CAD build for the part. Positions are in the model's coordinates, mm. A direction names the side the tool comes from. Give positions to 0.01 mm unless a question says otherwise; leave off trailing zeros. Loops run counter-clockwise (first coordinate to the right, second up) from the corner with the lowest first, then second, coordinate; pieces in that order, holes last. Notation, with made-up numbers: (-10, 64) -> (-4, 64) arc R24 cw to (-4, 79) -> close; hole circle Ø10 at (-2.5, -34). An arc over 180 degrees is marked (long way). Use one line per item in the form item = value.
Autodesk Inventor part; units mm, degrees
ref_plane "YZ Plane" through (0, 0, 0) normal (1, 0, 0) x (0, 1, 0)
ref_plane "XZ Plane" through (0, 0, 0) normal (0, 1, 0) x (-1, 0, 0)
ref_plane "XY Plane" through (0, 0, 0) normal (0, 0, 1) x (1, 0, 0)
sketch "MainSketch1" plane through (0, 0, 0) normal (0, 0, 1) x (1, 0, 0)
  line L0 (0, 0) -> (86.36, 0)
  line L1 (86.36, 0) -> (86.36, 25.4)
  line L2 (86.36, 25.4) -> (76.2, 25.4)
  line L3 (76.2, 25.4) -> (76.2, 19.05)
  line L4 (76.2, 19.05) -> (67.31, 19.05)
  line L5 (67.31, 19.05) -> (67.31, 25.4)
  line L6 (67.31, 25.4) -> (19.05, 25.4)
  line L7 (19.05, 25.4) -> (19.05, 19.05)
  line L8 (19.05, 19.05) -> (10.16, 19.05)
  line L9 (10.16, 19.05) -> (10.16, 25.4)
  line L10 (10.16, 25.4) -> (0, 25.4)
  line L11 (0, 25.4) -> (0, 0)
  line L12 (381, 0) -> (381, 63.5) construction
  dimension "d0" = 86.36
  dimension "d1" = 10.16
  dimension "d2" = 19.05
  dimension "d3" = 67.31
  dimension "d4" = 76.2
  dimension "d5" = 19.05
  dimension "d6" = 25.4
  dimension "d7" = 25.4
  dimension "d8" = 19.05
  dimension "d9" = 25.4
  dimension "d10" = 381
  dimension "d30" = 63.5
revolve "MainRevolution1" add sketch "MainSketch1" angle 45 about axis through (381, 0, 0) along (0, 1, 0)
sketch "HeadSketch" plane through (19.05, 25.4, 0) normal (0, 1, 0) x (1, 0, 0)
  line L0 (48.26, 0) -> (0, 0)
  arc A0 (31.75, 9.3356) -> (16.51, 9.3356) centre (24.13, 25.4) ccw
  arc A1 (-19.05, 0) -> (92.5423, -269.4077) centre (361.95, 0) ccw
  arc A2 (67.31, 0) -> (153.6081, -208.3419) centre (361.95, 0) ccw
  line L1 (-8.89, 0) -> (-19.05, 0)
  line L2 (67.31, 0) -> (57.15, 0)
  line L3 (57.15, 0) -> (48.26, 0)
  line L4 (0, 0) -> (-8.89, 0)
  line L5 (92.5423, -269.4077) -> (99.7265, -262.2235)
  line L6 (99.7265, -262.2235) -> (106.0127, -255.9373)
  line L7 (140.1377, -221.8123) -> (146.4239, -215.5261)
  line L8 (146.4239, -215.5261) -> (153.6081, -208.3419)
  line L9 (16.51, 0) -> (31.75, 0)
  line L10 (31.75, 0) -> (31.75, 9.3356)
  line L11 (16.51, 9.3356) -> (16.51, 0)
  line L12 (106.0127, -255.9373) -> (140.1377, -221.8123)
  arc A3 (123.0945, -227.2198) -> (111.4202, -238.8941) centre (105.1174, -220.917) ccw
  line L13 (128.9124, -233.0376) -> (123.0945, -227.2198)
  line L14 (111.4202, -238.8941) -> (117.238, -244.712)
  line L15 (117.238, -244.712) -> (128.9124, -233.0376)
  line L16 (123.0945, -227.2198) -> (111.4202, -238.8941) construction
  line L17 (105.1174, -220.917) -> (123.0752, -238.8748) construction
  point P0 (24.13, 0)
  dimension "d12" = 43.18
  dimension "d13" = 25.4
  dimension "d14" = 35.56
  dimension "d15" = 15.24
  dimension "d16" = 43.18
  dimension "d26" = 38.1
  dimension "d27" = 16.51
  dimension "d32" = 90
  dimension "d33" = 90
  dimension "d34" = 17.9578
extrude "TopHeadExtrusion1" add sketch "HeadSketch" against normal blind 25.4 contours L0 L11 A0 L10
extrude "BottomHeadCut" cut sketch "HeadSketch" against normal through all contours L12 L14 A3 L13
fillet "NeckFillet" radius 4.826 4 edges at (50.8, 12.7, -9.3356) (35.56, 12.7, -9.3356) (142.1445, 12.7, 227.2198) (130.4702, 12.7, 238.8941)
properties part number "CurvedTrack"
1. Drop flat-ended pins along their axis: P1, Ø3, axis at y = 3, z = 156, coming from the -X side; P2, Ø7, axis at y = 9, z = -4.5, coming from the +X side; P3, Ø7, axis at y = 6.5, z = -1.5, coming from the -X side; P4, Ø8, axis at x = 152.5, y = 16.5, coming from the -Z side. Give the stop position or say it passes through.
Result sheet:
P1 = 32.73
P2 = 51.03
P3 = 0
P4 = 180.99
2. Mould opens along Z. For faces 5 (the flat face through (68, 13, 0)), 6 (the cylindrical face through (108.172, 12.878, 111.256)), 7 (the flat face through (69, 25.4, 107)) say: pulls with the +Z half, pulls with the -Z half, needs draft (parallel to the pull), parting line crosses it, or undercut.
Result sheet:
face_5 = undercut
face_6 = pulls with the -Z half
face_7 = needs draft
3. Cut at C-C, the plane z = 177. Write the cut outline in (x, y), then the cut area to 3 significant figures.
Result sheet:
outline = (43.61, 0) -> (145.45, 0) -> (145.45, 25.4) -> (132.86, 25.4) -> (132.86, 19.05) -> (122.02, 19.05) -> (122.02, 25.4) -> (65.28, 25.4) -> (65.28, 19.05) -> (55.13, 19.05) -> (55.13, 25.4) -> (43.61, 25.4) -> close
area = 2,450 mm^2
4. Cut at B-B, the plane y = 22. Write the cut outline in (x, z).
Result sheet:
outline = (0, 0) -> (10.16, 0) arc R370.84 cw to (118.78, 262.22) -> (111.59, 269.41) arc R381 ccw to start; (19.05, 0) -> (35.56, 0) -> (35.56, -6.53) arc R4.83 cw to (33.39, -10.56) arc R17.78 ccw (long way) to (52.97, -10.56) arc R4.83 cw to (50.8, -6.53) -> (50.8, 0) -> (67.31, 0) arc R313.69 cw to (159.19, 221.81) -> (147.96, 233.04) -> (144.13, 229.2) arc R4.83 ccw to (142.82, 224.81) arc R19.05 cw (long way) to (128.06, 239.57) arc R4.83 ccw to (132.45, 240.88) -> (136.29, 244.71) -> (125.06, 255.94) arc R361.95 ccw to start; (76.2, 0) -> (86.36, 0) arc R294.64 cw to (172.66, 208.34) -> (165.47, 215.53) arc R304.8 ccw to start
5. Cut at D-D, the plane x = 98. Write the cut outline in (y, z), then the cut area to 3 significant figures.
Result sheet:
outline = (0, 82) -> (25.4, 82) -> (25.4, 113.2) -> (19.05, 113.2) -> (19.05, 135.32) -> (25.4, 135.32) -> (25.4, 225.65) -> (19.05, 225.65) -> (19.05, 239.65) -> (25.4, 239.65) -> (25.4, 255.09) -> (0, 255.09) -> close
area = 4,170 mm^2
6. Drill centre lines: line 1 (X direction, y = 19.75, z = 181.5); line 2 (Y direction, x = 12, z = 35.5); line 3 (X direction, y = 19.5, z = 234). Where is each one in solid material? Low to high.
Result sheet:
line_1 = 46.01 to 57.61, 67.85 to 125.15, 136.13 to 148.9
line_2 = 0 to 19.05
line_3 = 80.33 to 93.31, 104.86 to 110.32
7. Cut at A-A, the plane x = 115.5. Write the cut outline in (y, z), then the cut area to 3 significant figures.
Result sheet:
outline = (0, 127.76) -> (25.4, 127.76) -> (25.4, 149.71) -> (19.05, 149.71) -> (19.05, 167.07) -> (25.4, 167.07) -> (25.4, 203.95) -> (0, 203.95) -> close; (0, 237.88) -> (25.4, 237.88) -> (25.4, 246) -> (19.05, 246) -> (19.05, 258.91) -> (25.4, 258.91) -> (25.4, 265.5) -> (0, 265.5) -> close
area = 2,440 mm^2
8. Tool access for faces 1 (the flat face through (50.8, 13, -3)), 2 (the cylindrical face through (100.047, 22.181, 118.188)), 3 (the cylindrical face through (111.19, 12.88, 206.97)), 4 (the flat face through (18, 13, 0)): list every direction of +Z, -Z, +X, -X, +Y, -Y with a clear straight run to the whole face (end or side of a thin tool).
Result sheet:
face_1 = +X, +Y, -Y
face_2 = +Y
face_3 = +Y, -Y
face_4 = -X, +Y, -Y
